from build123d import *

# Parameters (mm, degrees)
SKETCH2_W                                           = 152.4
SKETCH2_H                                           = 984.25
BOSS_EXTRUDE1_DEPTH                                 = 9.525
SKETCH4_W                                           = 142.875
SKETCH4_H                                           = 984.25
BOSS_EXTRUDE2_DEPTH                                 = 9.525
SKETCH5_R                                           = 3.5687
CUT_EXTRUDE1_DEPTH                                  = 9.525
SKETCH6_R                                           = 3.5687
CUT_EXTRUDE2_DEPTH                                  = 9.525
CSK_FOR_1_4_FLAT_HEAD_MACHINE_SCREW1_D              = 6.7564
CSK_FOR_1_4_FLAT_HEAD_MACHINE_SCREW1_CSINK_D        = 15.5273756
CSK_FOR_1_4_FLAT_HEAD_MACHINE_SCREW1_CSINK_ANGLE    = 82
CSK_FOR_1_4_FLAT_HEAD_MACHINE_SCREW2_D              = 6.7564
CSK_FOR_1_4_FLAT_HEAD_MACHINE_SCREW2_CSINK_D        = 15.5273756
CSK_FOR_1_4_FLAT_HEAD_MACHINE_SCREW2_CSINK_ANGLE    = 82
CSK_FOR_1_4_FLAT_HEAD_MACHINE_SCREW_100_D           = 6.7564
CSK_FOR_1_4_FLAT_HEAD_MACHINE_SCREW_100_CSINK_D     = 16.510254
CSK_FOR_1_4_FLAT_HEAD_MACHINE_SCREW_100_CSINK_ANGLE = 100
CSK_FOR_1_4_FLAT_HEAD_MACHINE_SCREW5_D              = 6.7564
CSK_FOR_1_4_FLAT_HEAD_MACHINE_SCREW5_CSINK_D        = 15.5273756
CSK_FOR_1_4_FLAT_HEAD_MACHINE_SCREW5_CSINK_ANGLE    = 82
CSK_FOR_1_4_FLAT_HEAD_MACHINE_SCREW6_D              = 6.7564
CSK_FOR_1_4_FLAT_HEAD_MACHINE_SCREW6_CSINK_D        = 15.5273756
CSK_FOR_1_4_FLAT_HEAD_MACHINE_SCREW6_CSINK_ANGLE    = 82
CSK_FOR_1_4_FLAT_HEAD_MACHINE_SCREW7_D              = 6.7564
CSK_FOR_1_4_FLAT_HEAD_MACHINE_SCREW7_CSINK_D        = 15.5273756
CSK_FOR_1_4_FLAT_HEAD_MACHINE_SCREW7_CSINK_ANGLE    = 82
CSK_FOR_1_4_FLAT_HEAD_MACHINE_SCREW8_D              = 6.7564
CSK_FOR_1_4_FLAT_HEAD_MACHINE_SCREW8_CSINK_D        = 15.5273756
CSK_FOR_1_4_FLAT_HEAD_MACHINE_SCREW8_CSINK_ANGLE    = 82
CSK_FOR_1_4_FLAT_HEAD_MACHINE_SCREW4_D              = 6.7564
CSK_FOR_1_4_FLAT_HEAD_MACHINE_SCREW4_CSINK_D        = 15.5273756
CSK_FOR_1_4_FLAT_HEAD_MACHINE_SCREW4_CSINK_ANGLE    = 82


with BuildPart() as part:
    # Sketch2 → Boss-Extrude1 (new body)
    with BuildSketch(Plane.XY):
        with Locations((7.535690004, -455.883176253)):
            Rectangle(SKETCH2_W, SKETCH2_H)
    extrude(amount=BOSS_EXTRUDE1_DEPTH)

    # Sketch4 → Boss-Extrude2 (add)
    with BuildSketch(Plane.ZY.offset(68.664309996)):
        with Locations((-71.4375, -455.883176253)):
            Rectangle(SKETCH4_W, SKETCH4_H)
    extrude(amount=-BOSS_EXTRUDE2_DEPTH)

    # Sketch5 → Cut-Extrude1 (cut)
    with BuildSketch(Plane.ZY.offset(68.664309996)):
        with Locations((-104.775, -151.083176253)):
            Circle(SKETCH5_R)
        with Locations((-104.775, -354.283176253)):
            Circle(SKETCH5_R)
        with Locations((-104.775, -557.483176253)):
            Circle(SKETCH5_R)
        with Locations((-104.775, -760.683176253)):
            Circle(SKETCH5_R)
    extrude(amount=-CUT_EXTRUDE1_DEPTH, mode=Mode.SUBTRACT)

    # Sketch6 → Cut-Extrude2 (cut)
    with BuildSketch(Plane.XY.offset(9.525)):
        with Locations((45.635690004, -151.083176253)):
            Circle(SKETCH6_R)
        with Locations((45.635690004, -354.283176253)):
            Circle(SKETCH6_R)
        with Locations((45.635690004, -557.483176253)):
            Circle(SKETCH6_R)
        with Locations((45.635690004, -760.683176253)):
            Circle(SKETCH6_R)
    extrude(amount=-CUT_EXTRUDE2_DEPTH, mode=Mode.SUBTRACT)

    # CSK for 1/4 Flat Head Machine Screw1 (through all)
    with Locations(Plane(origin=(-59.139309996, -151.083176253, -104.775), x_dir=(0, 0, 1), z_dir=(1, 0, 0))):
        with Locations((0, 0)):
            CounterSinkHole(CSK_FOR_1_4_FLAT_HEAD_MACHINE_SCREW1_D / 2, CSK_FOR_1_4_FLAT_HEAD_MACHINE_SCREW1_CSINK_D / 2, counter_sink_angle=CSK_FOR_1_4_FLAT_HEAD_MACHINE_SCREW1_CSINK_ANGLE)

    # CSK for 1/4 Flat Head Machine Screw2 (through all)
    with Locations(Plane(origin=(-59.139309996, -354.283176253, -104.775), x_dir=(0, 0, 1), z_dir=(1, 0, 0))):
        with Locations((0, 0)):
            CounterSinkHole(CSK_FOR_1_4_FLAT_HEAD_MACHINE_SCREW2_D / 2, CSK_FOR_1_4_FLAT_HEAD_MACHINE_SCREW2_CSINK_D / 2, counter_sink_angle=CSK_FOR_1_4_FLAT_HEAD_MACHINE_SCREW2_CSINK_ANGLE)

    # CSK for 1/4 Flat Head Machine Screw (100)4 (through all)
    with Locations(Plane(origin=(-59.139309996, -760.683176253, -104.775), x_dir=(0, 0, 1), z_dir=(1, 0, 0))):
        with Locations((0, 0)):
            CounterSinkHole(CSK_FOR_1_4_FLAT_HEAD_MACHINE_SCREW_100_D / 2, CSK_FOR_1_4_FLAT_HEAD_MACHINE_SCREW_100_CSINK_D / 2, counter_sink_angle=CSK_FOR_1_4_FLAT_HEAD_MACHINE_SCREW_100_CSINK_ANGLE)

    # CSK for 1/4 Flat Head Machine Screw5 (through all)
    with Locations(Plane(origin=(45.635690004, -151.083176253, 0), x_dir=(-1, 0, 0), z_dir=(0, 0, -1))):
        with Locations((0, 0)):
            CounterSinkHole(CSK_FOR_1_4_FLAT_HEAD_MACHINE_SCREW5_D / 2, CSK_FOR_1_4_FLAT_HEAD_MACHINE_SCREW5_CSINK_D / 2, counter_sink_angle=CSK_FOR_1_4_FLAT_HEAD_MACHINE_SCREW5_CSINK_ANGLE)

    # CSK for 1/4 Flat Head Machine Screw6 (through all)
    with Locations(Plane(origin=(45.635690004, -354.283176253, 0), x_dir=(-1, 0, 0), z_dir=(0, 0, -1))):
        with Locations((0, 0)):
            CounterSinkHole(CSK_FOR_1_4_FLAT_HEAD_MACHINE_SCREW6_D / 2, CSK_FOR_1_4_FLAT_HEAD_MACHINE_SCREW6_CSINK_D / 2, counter_sink_angle=CSK_FOR_1_4_FLAT_HEAD_MACHINE_SCREW6_CSINK_ANGLE)

    # CSK for 1/4 Flat Head Machine Screw7 (through all)
    with Locations(Plane(origin=(45.635690004, -557.483176253, 0), x_dir=(-1, 0, 0), z_dir=(0, 0, -1))):
        with Locations((0, 0)):
            CounterSinkHole(CSK_FOR_1_4_FLAT_HEAD_MACHINE_SCREW7_D / 2, CSK_FOR_1_4_FLAT_HEAD_MACHINE_SCREW7_CSINK_D / 2, counter_sink_angle=CSK_FOR_1_4_FLAT_HEAD_MACHINE_SCREW7_CSINK_ANGLE)

    # CSK for 1/4 Flat Head Machine Screw8 (through all)
    with Locations(Plane(origin=(45.635690004, -760.683176253, 0), x_dir=(-1, 0, 0), z_dir=(0, 0, -1))):
        with Locations((0, 0)):
            CounterSinkHole(CSK_FOR_1_4_FLAT_HEAD_MACHINE_SCREW8_D / 2, CSK_FOR_1_4_FLAT_HEAD_MACHINE_SCREW8_CSINK_D / 2, counter_sink_angle=CSK_FOR_1_4_FLAT_HEAD_MACHINE_SCREW8_CSINK_ANGLE)

    # CSK for 1/4 Flat Head Machine Screw4 (through all)
    with Locations(Plane(origin=(-59.139309996, -557.483176253, -104.775), x_dir=(0, 0, 1), z_dir=(1, 0, 0))):
        with Locations((0, 0)):
            CounterSinkHole(CSK_FOR_1_4_FLAT_HEAD_MACHINE_SCREW4_D / 2, CSK_FOR_1_4_FLAT_HEAD_MACHINE_SCREW4_CSINK_D / 2, counter_sink_angle=CSK_FOR_1_4_FLAT_HEAD_MACHINE_SCREW4_CSINK_ANGLE)


solid = part.part
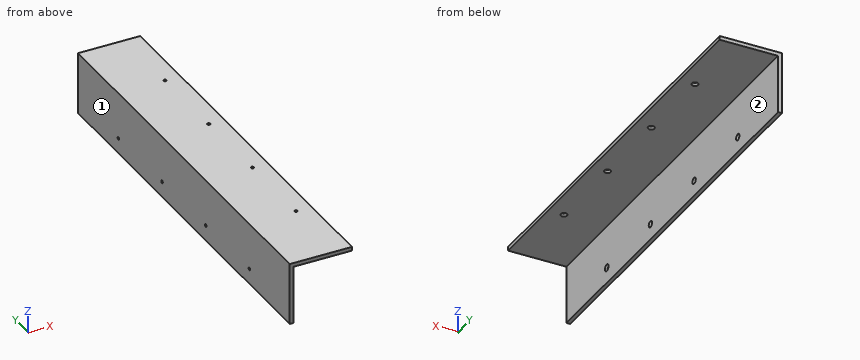
Source: CAD feature listing. Evaluate the final solid. Frame: model axes, mm. Face numbers are marked on the shaded views. A direction names the side the tool comes from. Give positions to 0.01 mm unless a question says otherwise; leave off trailing zeros. Write each loop counter-clockwise with the first axis right and the second up, starting at its lowest first coordinate (ties: lowest second). Pieces come first, ordered by that corner, then holes. Notation, with made-up numbers: (-6, -17.75) - (24, -17.75) arc R19 ccw to (24, 12.25) - close; hole circle Ø3 at (-18, 29.25). An arc over 180 degrees is marked (long way). Write item = value, one per line. Start each with the question number.
Q1. Pin query (flat end, axial travel): pin 1 Ø11.5 at (x, y) = (45.64, -557.48) entering from -Z; pin 2 Ø3 at (x, y) = (-26.5, -620.5) entering from -Z; pin 3 Ø10 at (y, z) = (-607.5, -95) entering from +X. Return the tip coordinate at first contact, or that it passes through.
Q2. Cut plane C-C, the plane z = -17. Return loops of the section in (x, y).
Q3. Cut plane B-B, the plane x = -38.5. Return loops of the section in (y, z) (3 decimals).
Q4. Cut plane A-A, the plane y = -289. Return loops of the section in (x, z) (3 decimals).
Q5. Material intervals for probe 1 along X at (y, z) = (-120, -74); probe 2 along Z at (x, y) = (-22, -37.5) (3 decimals), sorted ascending.
Q6. Reachability of the marked faces 1 and 2 from +Z, -Z, +X, -X, +Y, -Y: full face, straight path, thin tool, end or side. Return the list, or none.
Computed values:
q1.pin_1 = 2.31
q1.pin_2 = 0
q1.pin_3 = -59.14
q2.outline = (-68.66, -948.01) - (-59.14, -948.01) - (-59.14, 36.24) - (-68.66, 36.24) - close
q3.outline = (-948.008, 0) - (36.242, 0) - (36.242, 9.525) - (-948.008, 9.525) - close
q4.outline = (-68.664, -142.875) - (-59.139, -142.875) - (-59.139, 0) - (83.736, 0) - (83.736, 9.525) - (-68.664, 9.525) - close
q5.probe_1 = -68.66 to -59.14
q5.probe_2 = 0 to 9.525
q6.face_1 = +Z, -Z, -X, +Y, -Y
q6.face_2 = -Z, +X, +Y, -Y
